Verification items for the finished model (mm, model axes). A direction names the side the tool comes from. Coordinates: 2 decimals unless noted, no trailing zeros. Loops run counter-clockwise (first coordinate to the right, second up) from the corner with the lowest first, then second, coordinate; pieces in that order, holes last.
Q1. Access from +Z, -Z, +X, -X, +Y, -Y to the whole of each face (thin tool, end or side, straight path). Record for faces 1 (the face through (3.82, 10.42, 2.54)), 2 (the face through (3.5, 16, 2)), 3 (the face through (4.5, -19, 2)), 4 (the face through (-8.5, 17, 2)).
Q2. Sectioned sample at A-A (y = 0). Enter the section's corners in (x, z), then the cut area to 3 significant figures.
Q3. Material ranges on probe 1 along X at (y, z) = (0, 1.2); probe 2 along X at (y, z) = (15.5, 3.15); probe 3 along Y at (x, z) = (0, 3.35), recorded low to high.
Q4. Sectioned sample at D-D (y = 9). Enter the section's corners in (x, z), then the cut area to 3 significant figures.
Q5. Sectioned sample at B-B (z = 1.2). Enter the section's corners in (x, y), then the cut area to 3 significant figures.
Q6. Sectioned sample at C-C (x = 0). Enter the section's corners in (y, z), then the cut area to 3 significant figures.
Q7. Mould release check, pull along Y, two halves, no side actions. Record for faces 5 (the face through (8.5, 18, 2)), 6 (the face through (8.71, 13.42, 2.54)), 7 (the face through (-3.8, 10.45, 2.54)): +Y half, -Y half, draft (parallel to the pull), parting line (faces both ways), or undercut.
Q8. Go/stop test with flat-tipped pins: P1, Ø1.5, axis at y = 16, z = 1.5, coming from the -X side; P2, Ø2, axis at x = 4.5, y = -7, coming from the -Z side (3 decimals); P3, Ø1.5, axis at y = -3, z = 2.5, coming from the -X side; P4, Ø1.5, axis at y = 17, z = 2, coming from the +X side. Record where each tip stops, or that it passes through.
```python
from build123d import *

# Parameters (mm, degrees)
BOSS_EXTRUDE1_DEPTH = 5
FILLET1_R           = 2


with BuildPart() as part:
    # Sketch1 → Boss-Extrude1 (new body)
    with BuildSketch(Plane.XY):
        with BuildLine():
            Line((3.5, 22.759430606), (8.5, 22.759430606))
            Line((8.5, 22.759430606), (8.5, 13.259430606))
            ThreePointArc((8.5, 13.259430606), (15.595562994, -2.200207922), (4.5, -15.093458848))
            Line((4.5, -15.093458848), (4.5, -24.093458848))
            Line((4.5, -24.093458848), (-4.5, -24.093458848))
            Line((-4.5, -24.093458848), (-4.5, -15.093458848))
            ThreePointArc((-4.5, -15.093458848), (-15.595562994, -2.200207922), (-8.5, 13.259430606))
            Line((-8.5, 13.259430606), (-8.5, 22.759430606))
            Line((-8.5, 22.759430606), (-3.5, 22.759430606))
            Line((-3.5, 22.759430606), (-3.5, 10.164275675))
            ThreePointArc((-3.5, 10.164275675), (0, -10.75), (3.5, 10.164275675))
            Line((3.5, 10.164275675), (3.5, 22.759430606))
        make_face()
    extrude(amount=BOSS_EXTRUDE1_DEPTH)

    # Fillet1
    fillet1_edges = [part.edges().sort_by_distance(p)[0] for p in [
        (4.5, -15.093458848, 2.5),
        (4.5, -24.093458848, 2.5),
        (-4.5, -24.093458848, 2.5),
        (-4.5, -15.093458848, 2.5),
        (-8.5, 13.259430606, 2.5),
        (-8.5, 22.759430606, 2.5),
        (-3.5, 22.759430606, 2.5),
        (-3.5, 10.164275675, 2.5),
        (3.5, 10.164275675, 2.5),
        (3.5, 22.759430606, 2.5),
        (8.5, 22.759430606, 2.5),
        (8.5, 13.259430606, 2.5),
    ]]
    fillet(fillet1_edges, radius=FILLET1_R)


solid = part.part
```
Geometry check:
1. face 1: +Z, -Z
1. face 2: +Z, -Z, +Y
1. face 3: +Z, -Z, +X, -Y
1. face 4: +Z, -Z, -X, +Y
2. outline: (-15.75, 0) - (-10.75, 0) - (-10.75, 5) - (-15.75, 5) - close; (10.75, 0) - (15.75, 0) - (15.75, 5) - (10.75, 5) - close
2. area: 50.0 mm2
3. probe 1: x = -15.75 to -10.75, 10.75 to 15.75
3. probe 2: x = -8.5 to -3.5, 3.5 to 8.5
3. probe 3: y = -24.09 to -10.75
4. outline: (-12.93, 0) - (-5.88, 0) - (-5.88, 5) - (-12.93, 5) - close; (5.88, 0) - (12.93, 0) - (12.93, 5) - (5.88, 5) - close
4. area: 70.5 mm2
5. outline: (-9.32, 12.7) arc R15.75 ccw to (-5.77, -14.66) arc R2 cw to (-4.5, -16.52) - (-4.5, -22.09) arc R2 ccw to (-2.5, -24.09) - (2.5, -24.09) arc R2 ccw to (4.5, -22.09) - (4.5, -16.52) arc R2 cw to (5.77, -14.66) arc R15.75 ccw to (9.32, 12.7) arc R2 cw to (8.5, 14.31) - (8.5, 20.76) arc R2 ccw to (6.5, 22.76) - (5.5, 22.76) arc R2 ccw to (3.5, 20.76) - (3.5, 11.5) arc R2 ccw to (4.64, 9.7) arc R10.75 cw (long way) to (-4.64, 9.7) arc R2 ccw to (-3.5, 11.5) - (-3.5, 20.76) arc R2 ccw to (-5.5, 22.76) - (-6.5, 22.76) arc R2 ccw to (-8.5, 20.76) - (-8.5, 14.31) arc R2 cw to start
5. area: 536 mm2
6. outline: (-24.09, 0) - (-10.75, 0) - (-10.75, 5) - (-24.09, 5) - close
6. area: 66.7 mm2
7. face 5: draft
7. face 6: +Y half
7. face 7: undercut
8. P1: stops at x = -8.5
8. P2: passes through
8. P3: stops at x = -15.59
8. P4: stops at x = 8.5
